Check sheet for the modelled part. Datum: model origin and axes. Units: mm. A direction names the side the tool comes from. Round coordinates to 2 decimals unless told otherwise and drop trailing zeros. Loops run counter-clockwise (first coordinate to the right, second up) from the corner with the lowest first, then second, coordinate; pieces in that order, holes last. Notation, with made-up numbers: (-17, 50.5) -> (39, 50.5) arc R32 cw to (39, 89.5) -> close; hole circle Ø9 at (86, 73). An arc over 180 degrees is marked (long way). Return JSON: item names as keys, results as strings.
from build123d import *

# Parameters (mm, degrees)
EXTRUDE_1_DEPTH     = 4.58
SKETCH_2_W          = 0.46
SKETCH_2_H          = 0.38
EXTRUDE_2_DEPTH     = 5
SKETCH_3_R          = 0.6
CUT_EXTRUDE_1_DEPTH = 0.2


with BuildPart() as part:
    # Sketch 1 → Extrude 1 (new body)
    with BuildSketch(Plane.XY):
        with BuildLine():
            Line((-2.276312808, 0.25), (2.276312808, 0.25))
            ThreePointArc((2.276312808, 0.25), (0, -2.29), (-2.276312808, 0.25))
        make_face()
        Polygon((1.8, 1.27), (2.276312808, 0.25), (-2.276312808, 0.25), (-1.8, 1.27), align=None)
    extrude(amount=EXTRUDE_1_DEPTH)

    # Sketch 2 → Extrude 2 (add)
    with BuildSketch(Plane(origin=(0, 0, 0), x_dir=(-1, 0, 0), z_dir=(0, 0, -1))):
        with Locations((0.006718678, 0.19)):
            Rectangle(SKETCH_2_W, SKETCH_2_H)
        with Locations((1.276718678, 0.19)):
            Rectangle(SKETCH_2_W, SKETCH_2_H)
        with Locations((-1.263281322, 0.19)):
            Rectangle(SKETCH_2_W, SKETCH_2_H)
    extrude(amount=EXTRUDE_2_DEPTH)

    # Sketch 3 → Cut-Extrude 1 (cut)
    with BuildSketch(Plane(origin=(0, -2.29, 0), x_dir=(-1, 0, 0), z_dir=(0, 1, 0))):
        with Locations(Location((0, 2.220906824, 0), (0, 0, 270))):
            Circle(SKETCH_3_R)
    extrude(amount=CUT_EXTRUDE_1_DEPTH, mode=Mode.SUBTRACT)


solid = part.part
Q1. Tool access check on faces 1 (the flat face through (0, -2.09, 2)), 2 (the flat face through (0, 0, 4.58)). Record the directions out of +Z, -Z, +X, -X, +Y, -Y that give a thin tool (end or side, any length) a straight path to the whole face; none if there is none.
Results list:
{"face 1": "-Y", "face 2": "+Z, +X, -X, +Y, -Y"}
Q2. Section check B-B (x = 0). Record the boundary of the cut face in (y, z), then the cut area to 3 significant figures.
Results list:
{"outline": "(-2.29, 0) -> (0, 0) -> (0, -5) -> (0.38, -5) -> (0.38, 0) -> (1.27, 0) -> (1.27, 4.58) -> (-2.29, 4.58) -> (-2.29, 2.82) -> (-2.09, 2.82) -> (-2.09, 1.62) -> (-2.29, 1.62) -> close", "area": "18.0 mm^2"}
Q3. Go/stop test with flat-tipped pins: pin 1 (1.1 mm diameter, centred on x = -0.5, y = 0, fed in from -Z); pin 2 (1.5 mm diameter, centred on x = 0, z = -1, fed in from +Y); pin 3 (0.5 mm diameter, centred on x = -1, z = -2, fed in from -Y). Record where each tip stops, or that it passes through.
Results list:
{"pin 1": "z = -5", "pin 2": "y = 0.38", "pin 3": "y = 0"}
Q4. Section check D-D (y = 0.1). Record the boundary of the cut face in (x, z), then the cut area to 3 significant figures.
Results list:
{"outline": "(-2.29, 0) -> (-1.51, 0) -> (-1.51, -5) -> (-1.05, -5) -> (-1.05, 0) -> (-0.24, 0) -> (-0.24, -5) -> (0.22, -5) -> (0.22, 0) -> (1.03, 0) -> (1.03, -5) -> (1.49, -5) -> (1.49, 0) -> (2.29, 0) -> (2.29, 4.58) -> (-2.29, 4.58) -> close", "area": "27.9 mm^2"}
Q5. Section check C-C (z = 1.75). Record the boundary of the cut face in (x, y), then the cut area to 3 significant figures.
Results list:
{"outline": "(-2.28, 0.25) arc R2.29 ccw to (-0.37, -2.26) -> (-0.37, -2.09) -> (0.37, -2.09) -> (0.37, -2.26) arc R2.29 ccw to (2.28, 0.25) -> (1.8, 1.27) -> (-1.8, 1.27) -> close", "area": "13.4 mm^2"}
Q6. Section check A-A (z = -2.75). Record the boundary of the cut face in (x, y), then the cut area to 3 significant figures.
Results list:
{"outline": "(-1.51, 0) -> (-1.05, 0) -> (-1.05, 0.38) -> (-1.51, 0.38) -> close; (-0.24, 0) -> (0.22, 0) -> (0.22, 0.38) -> (-0.24, 0.38) -> close; (1.03, 0) -> (1.49, 0) -> (1.49, 0.38) -> (1.03, 0.38) -> close", "area": "0.524 mm^2"}
Q7. Material ranges on line 1 (Z direction, x = 2, y = 0.15); line 2 (Y direction, x = 1.35, z = -3.75); line 3 (X direction, y = -0.15, z = 2.25), recorded low to high.
Results list:
{"line 1": "0 to 4.58", "line 2": "0 to 0.38", "line 3": "-2.29 to 2.29"}
